Design review of the part built by this model. Coordinates are the model's own, in mm. Face numbers are marked on the shaded views. A direction names the side the tool comes from. Coordinates: 2 decimals unless noted, no trailing zeros. Loops run counter-clockwise (first coordinate to the right, second up) from the corner with the lowest first, then second, coordinate; pieces in that order, holes last. Notation, with made-up numbers: M 45.25,26.25 L 71.25,26.25 A24 cw 71.25,49.25 Z; hole C 62.25,84.25 d8. An arc over 180 degrees is marked long. Answer as a JSON object with one key per item and string values. Group by question number.
1. Insertion check: pin 1 (1.7 mm diameter, centred on y = 4.5, z = -0.5, fed in from +X); pin 2 (0.9 mm diameter, centred on x = -0.5, z = 1, fed in from -Y); pin 3 (6 mm diameter, centred on y = -1.5, z = 0, fed in from +X); pin 4 (1 mm diameter, centred on x = -2, z = 4, fed in from -Y). Each pin has a flat end and moves straight along its axis. Give the tip position at first contact, or say it passes through.
2. Machinability: for the marked faces 1, 2 and 3, which of the approach directions +Z, -Z, +X, -X, +Y, -Y give a long, thin tool a straight path to every point of the face, cutting with its end or side? Answer none if there is none.
3. Draft analysis for pull direction Z (two halves, no side actions). For the marked faces 4, 5 and 6, state which applies: +Z half, -Z half, draft (parallel to the pull), parting line (faces both ways), or undercut.
4. To check wall thickness, follow probe 1 along Z at (x, y) = (-2.1, 0); probe 2 along Z at (x, y) = (-3.4, 1); probe 3 along Y at (x, z) = (-0.6, 2.5). State the ranges of each line that lie inside material, in increasing order.
5. Consider section D-D (y = -4). State the section outline as (x, z) points, then the cut area to 3 significant figures.
6. Consider section C-C (x = -2.95). State the section outline as (y, z) points.
7. Consider section A-A (z = 0). State the section outline as (x, y) points, then the cut area to 3 significant figures.
8. Consider section B-B (y = 0). State the section outline as (x, z) points.
Autodesk Inventor part; units mm, degrees
ref_plane "nut_XY" through (0, 0, 0) normal (1, 0, 0) x (0, 0, -1)
ref_plane "nut_YZ" through (0, 0, 0) normal (0, 0, -1) x (0, 1, 0)
ref_plane "nut_ZX" through (0, 0, 0) normal (0, 1, 0) x (1, 0, 0)
sketch "Sketch_4" plane through (0, 0, 0) normal (0, 0, 1) x (1, 0, 0)
  line L0 (-4.1, 2.9) -> (-4.1, -2.9)
  line L1 (-4.1, -2.9) -> (-0.8, -5)
  line L2 (-0.8, -5) -> (-0.8, -2.9)
  line L3 (-0.8, -2.9) -> (0, -2.9)
  line L4 (0, -2.9) -> (0, 2.9)
  line L5 (0, 2.9) -> (-0.8, 2.9)
  line L6 (-0.8, 2.9) -> (-0.8, 5)
  line L7 (-0.8, 5) -> (-4.1, 2.9)
extrude "Extrusion1" add sketch "Sketch_4" along normal mid plane 10
sketch "Sketch_5" plane through (0, 0, 0) normal (0, 0, 1) x (1, 0, 0)
  line L0 (0, 0) -> (-4.1, 0)
  line L1 (-4.1, 0) -> (-4.1, 2)
  line L2 (-4.1, 2) -> (-3.721, 1.621)
  line L3 (-3.721, 1.621) -> (-0.379, 1.621)
  line L4 (-0.379, 1.621) -> (0, 2)
  line L5 (0, 2) -> (0, 0)
  line L6 (0, 0) -> (-4.1, 0)
revolve "Revolution1" cut sketch "Sketch_5" angle 360 about axis through (0, 0, 0) along (1, 0, 0)
thread "Thread1"
ref_plane "nut_XY" through (0, 0, 0) normal (1, 0, 0) x (0, 0, -1)
ref_plane "nut_YZ" through (0, 0, 0) normal (0, 0, -1) x (0, 1, 0)
ref_plane "nut_ZX" through (0, 0, 0) normal (0, 1, 0) x (1, 0, 0)
ref_plane "to_bolt_XY" through (-4.1, 0, 0) normal (1, 0, 0) x (0, 0, -1)
ref_plane "to_bolt_YZ" through (-4.1, 0, 0) normal (0, 0, -1) x (0, 1, 0)
ref_plane "to_bolt_ZX" through (-4.1, 0, 0) normal (0, 1, 0) x (1, 0, 0)
ref_plane "to_frames_XY" through (-0.8, 0, 0) normal (1, 0, 0) x (0, 0, -1)
ref_plane "to_frames_YZ" through (-0.8, 0, 0) normal (0, 0, -1) x (0, 1, 0)
ref_plane "to_frames_ZX" through (-0.8, 0, 0) normal (0, 1, 0) x (1, 0, 0)
properties part number "HNTT5-4_1"
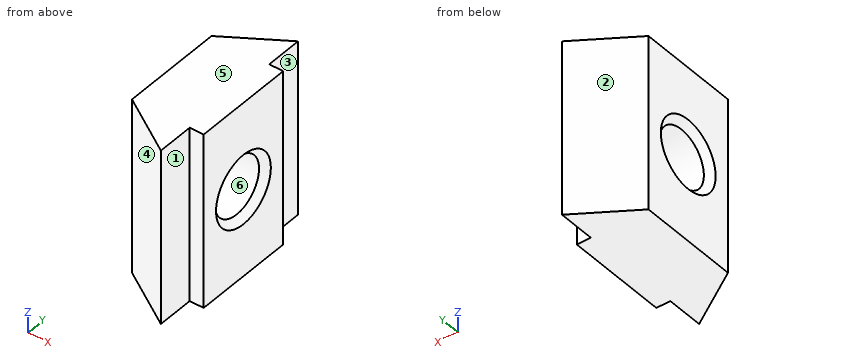
Findings below:
{
 "1": {"pin 1": "stops at x = -0.8", "pin 2": "stops at y = -5", "pin 3": "stops at x = 0", "pin 4": "stops at y = -4.55"},
 "2": {"face 1": "+Z, -Z, +X, -Y", "face 2": "+Z, -Z, -X, +Y", "face 3": "+Z, -Z, +X, +Y"},
 "3": {"face 4": "draft", "face 5": "+Z half", "face 6": "undercut"},
 "4": {"probe 1": "z = -5 to -1.62, 1.62 to 5", "probe 2": "z = -5 to -1.28, 1.28 to 5", "probe 3": "y = -2.9 to 2.9"},
 "5": {"outline": "M -2.37,-5 L -0.8,-5 L -0.8,5 L -2.37,5 Z", "area": "15.7 mm^2"},
 "6": {"outline": "M -3.63,-5 L 3.63,-5 L 3.63,5 L -3.63,5 Z; hole C 0,0 d3.24"},
 "7": {"outline": "M -4.1,-2.9 L -0.8,-5 L -0.8,-2.9 L 0,-2.9 L 0,-2 L -0.38,-1.62 L -3.72,-1.62 L -4.1,-2 Z; M -4.1,2 L -3.72,1.62 L -0.38,1.62 L 0,2 L 0,2.9 L -0.8,2.9 L -0.8,5 L -4.1,2.9 Z", "area": "17.1 mm^2"},
 "8": {"outline": "M -4.1,-5 L 0,-5 L 0,-2 L -0.38,-1.62 L -3.72,-1.62 L -4.1,-2 Z; M -4.1,2 L -3.72,1.62 L -0.38,1.62 L 0,2 L 0,5 L -4.1,5 Z"}
}
